```python
from build123d import *

# Parameters (mm, degrees)
EXTRUDE_1_OUTLINE_R   = 35
EXTRUDE_1_OUTLINE_R_2 = 1.55
EXTRUDE_1_OUTLINE_R_3 = 30.05
EXTRUDE_1_DEPTH       = 10
SKETCH_2_R            = 33.525
SKETCH_2_R_2          = 18.525
EXTRUDE_1_2_DEPTH     = 4
SKETCH_3_R            = 1.55
CUT_EXTRUDE_1_DEPTH   = 51.497524692
CUT_EXTRUDE_2_DEPTH   = 6
SKETCH_8_R            = 35
SKETCH_8_R_2          = 30.05
CUT_EXTRUDE_3_DEPTH   = 2
SKETCH_9_R            = 3
CUT_EXTRUDE_4_DEPTH   = 2
SKETCH_10_R           = 1.55
CUT_EXTRUDE_5_DEPTH   = 51.139804547
SKETCH_11_R           = 3
CUT_EXTRUDE_6_DEPTH   = 2
SKETCH_14_R           = 18.525
SKETCH_14_R_2         = 13.5
EXTRUDE_2_DEPTH       = 4
SKETCH_15_R           = 17.5
CUT_EXTRUDE_8_DEPTH   = 1.5
SKETCH_17_R           = 17.5
SKETCH_17_R_2         = 12.5
CUT_EXTRUDE_9_DEPTH   = 1
SKETCH1_R             = 13.5
SKETCH1_R_2           = 12
BOSS_EXTRUDE1_DEPTH   = 1
CUT_EXTRUDE1_START    = -2
SKETCH2_R             = 14
SKETCH2_R_2           = 13.5
CUT_EXTRUDE1_DEPTH    = 2
SKETCH3_R             = 14
SKETCH3_R_2           = 13.6
BOSS_EXTRUDE2_DEPTH   = 2
SKETCH5_R             = 12.5
SKETCH5_R_2           = 12
CUT_EXTRUDE3_DEPTH    = 50.922439844
SKETCH6_R             = 13
SKETCH6_R_2           = 12.5
CUT_EXTRUDE4_DEPTH    = 50.922439844
SKETCH7_R             = 17.5
SKETCH7_R_2           = 13.5
CUT_EXTRUDE5_DEPTH    = 0.5


# Read off the part's stored shape, not the designer's step: 凸台-拉伸1
with BuildPart() as part:
    # Extrude 1 outline → Extrude 1 (new body)
    with BuildSketch(Plane.XY):
        Circle(EXTRUDE_1_OUTLINE_R)
        with Locations((0, -32.5)):
            Circle(EXTRUDE_1_OUTLINE_R_2, mode=Mode.SUBTRACT)
        with Locations((-32.5, 0)):
            Circle(EXTRUDE_1_OUTLINE_R_2, mode=Mode.SUBTRACT)
        Circle(EXTRUDE_1_OUTLINE_R_3, mode=Mode.SUBTRACT)
        with Locations((32.5, 0)):
            Circle(EXTRUDE_1_OUTLINE_R_2, mode=Mode.SUBTRACT)
        with Locations((0, 32.5)):
            Circle(EXTRUDE_1_OUTLINE_R_2, mode=Mode.SUBTRACT)
    extrude(amount=EXTRUDE_1_DEPTH)

    # 草图2 → Extrude 1 2 (add)
    with BuildSketch(Plane.XY.offset(10)):
        Circle(SKETCH_2_R)
        Circle(SKETCH_2_R_2, mode=Mode.SUBTRACT)
    extrude(amount=-EXTRUDE_1_2_DEPTH)

    # 草图3 → 切除-拉伸1 (cut, through all)
    with BuildSketch(Plane(origin=(0, 0, 0), x_dir=(-1, 0, 0), z_dir=(0, 0, -1))):
        with Locations(Location((32.5, 0, 0), (0, 0, 180))):
            Circle(SKETCH_3_R)
        with Locations(Location((0, -32.5, 0), (0, 0, 180))):
            Circle(SKETCH_3_R)
        with Locations(Location((-32.5, 0, 0), (0, 0, 180))):
            Circle(SKETCH_3_R)
        with Locations(Location((0, 32.5, 0), (0, 0, 180))):
            Circle(SKETCH_3_R)
    extrude(amount=-CUT_EXTRUDE_1_DEPTH, mode=Mode.SUBTRACT)

    # 草图7 → 切除-拉伸2 (cut)
    with BuildSketch(Plane(origin=(0, 0, 0), x_dir=(-1, 0, 0), z_dir=(0, 0, -1))):
        with BuildLine():
            Line((15.025, 26.024063384), (17.5, 30.310889132))
            ThreePointArc((17.5, 30.310889132), (24.748737342, 24.748737342), (30.310889132, 17.5))
            Line((30.310889132, 17.5), (26.024063384, 15.025))
            ThreePointArc((26.024063384, 15.025), (21.248558775, 21.248558775), (15.025, 26.024063384))
        make_face()
    extrude(amount=-CUT_EXTRUDE_2_DEPTH, mode=Mode.SUBTRACT)

    # 草图8 → 切除-拉伸3 (cut)
    with BuildSketch(Plane(origin=(0, 0, 0), x_dir=(-1, 0, 0), z_dir=(0, 0, -1))):
        with Locations(Location((0, 0, 0), (0, 0, 30))):
            Circle(SKETCH_8_R)
        Circle(SKETCH_8_R_2, mode=Mode.SUBTRACT)
    extrude(amount=-CUT_EXTRUDE_3_DEPTH, mode=Mode.SUBTRACT)

    # 草图9 → 切除-拉伸4 (cut)
    with BuildSketch(Plane.XY.offset(10)):
        with Locations((0, 32.5)):
            Circle(SKETCH_9_R)
        with Locations((32.5, 0)):
            Circle(SKETCH_9_R)
        with Locations((0, -32.5)):
            Circle(SKETCH_9_R)
        with Locations((-32.5, 0)):
            Circle(SKETCH_9_R)
    extrude(amount=-CUT_EXTRUDE_4_DEPTH, mode=Mode.SUBTRACT)

    # 草图10 → 切除-拉伸5 (cut, through all)
    with BuildSketch(Plane.XY.offset(10)):
        with Locations((22.980970389, 22.980970389)):
            Circle(SKETCH_10_R)
        with Locations((22.980970389, -22.980970389)):
            Circle(SKETCH_10_R)
        with Locations((-22.980970389, -22.980970389)):
            Circle(SKETCH_10_R)
        with Locations((-22.980970389, 22.980970389)):
            Circle(SKETCH_10_R)
    extrude(amount=-CUT_EXTRUDE_5_DEPTH, mode=Mode.SUBTRACT)

    # 草图11 → 切除-拉伸6 (cut)
    with BuildSketch(Plane.XY.offset(10)):
        with Locations((22.980970389, 22.980970389)):
            Circle(SKETCH_11_R)
        with Locations((22.980970389, -22.980970389)):
            Circle(SKETCH_11_R)
        with Locations((-22.980970389, -22.980970389)):
            Circle(SKETCH_11_R)
        with Locations((-22.980970389, 22.980970389)):
            Circle(SKETCH_11_R)
    extrude(amount=-CUT_EXTRUDE_6_DEPTH, mode=Mode.SUBTRACT)

    # 草图14 → 凸台-拉伸2 (add)
    with BuildSketch(Plane.XY.offset(10)):
        Circle(SKETCH_14_R)
        Circle(SKETCH_14_R_2, mode=Mode.SUBTRACT)
    extrude(amount=-EXTRUDE_2_DEPTH)

    # 草图15 → 切除-拉伸8 (cut)
    with BuildSketch(Plane.XY.offset(10)):
        with BuildLine():
            ThreePointArc((21.378493867, 1.75), (0, 21.45), (-21.378493867, 1.75))
            Line((-21.378493866, 1.75), (-24.8, 1.75))
            Line((-24.8, 1.75), (-24.8, -1.75))
            Line((-24.8, -1.75), (-21.378493867, -1.75))
            ThreePointArc((-21.378493867, -1.75), (0, -21.45), (21.378493867, -1.75))
            Line((21.378493867, -1.75), (24.8, -1.75))
            Line((24.8, -1.75), (24.8, 1.75))
            Line((24.8, 1.75), (21.378493867, 1.75))
        make_face()
        Circle(SKETCH_15_R, mode=Mode.SUBTRACT)
    extrude(amount=-CUT_EXTRUDE_8_DEPTH, mode=Mode.SUBTRACT)

    # 草图17 → 切除-拉伸9 (cut)
    with BuildSketch(Plane.XY.offset(10)):
        Circle(SKETCH_17_R)
        Circle(SKETCH_17_R_2, mode=Mode.SUBTRACT)
    extrude(amount=-CUT_EXTRUDE_9_DEPTH, mode=Mode.SUBTRACT)

    # Sketch1 → Boss-Extrude1 (add)
    with BuildSketch(Plane.XY.offset(8.5)):
        Circle(SKETCH1_R)
        Circle(SKETCH1_R_2, mode=Mode.SUBTRACT)
    extrude(amount=-BOSS_EXTRUDE1_DEPTH)

    # Sketch2 → Cut-Extrude1 (cut)
    with BuildSketch(Plane(origin=(0, 0, 6), x_dir=(-1, 0, 0), z_dir=(0, 0, -1)).offset(CUT_EXTRUDE1_START)):
        Circle(SKETCH2_R)
        with Locations(Location((0, 0, 0), (0, 0, 180))):
            Circle(SKETCH2_R_2, mode=Mode.SUBTRACT)
    extrude(amount=CUT_EXTRUDE1_DEPTH, mode=Mode.SUBTRACT)

    # Sketch3 → Boss-Extrude2 (add)
    with BuildSketch(Plane(origin=(0, 0, 7.5), x_dir=(-1, 0, 0), z_dir=(0, 0, -1))):
        Circle(SKETCH3_R)
        Circle(SKETCH3_R_2, mode=Mode.SUBTRACT)
    extrude(amount=BOSS_EXTRUDE2_DEPTH)

    # Sketch5 → Cut-Extrude3 (cut, through all)
    with BuildSketch(Plane.XY.offset(8.5)):
        Circle(SKETCH5_R)
        Circle(SKETCH5_R_2, mode=Mode.SUBTRACT)
    extrude(amount=-CUT_EXTRUDE3_DEPTH, mode=Mode.SUBTRACT)

    # Sketch6 → Cut-Extrude4 (cut, through all)
    with BuildSketch(Plane.XY.offset(8.5)):
        Circle(SKETCH6_R)
        Circle(SKETCH6_R_2, mode=Mode.SUBTRACT)
    extrude(amount=-CUT_EXTRUDE4_DEPTH, mode=Mode.SUBTRACT)

    # Sketch7 → Cut-Extrude5 (cut)
    with BuildSketch(Plane.XY.offset(9)):
        Circle(SKETCH7_R)
        with Locations(Location((0, 0, 0), (0, 0, 180))):
            Circle(SKETCH7_R_2, mode=Mode.SUBTRACT)
    extrude(amount=-CUT_EXTRUDE5_DEPTH, mode=Mode.SUBTRACT)


solid = part.part
```
Source: CAD feature listing. Evaluate the final solid. Frame: model axes, mm. A direction names the side the tool comes from. Round coordinates to 2 decimals unless told otherwise and drop trailing zeros. Loops run counter-clockwise (first coordinate to the right, second up) from the corner with the lowest first, then second, coordinate; pieces in that order, holes last.
(1) Section query D-D (x = -19). Output: boundary loops of the cut face in (y, z), and give its area (3 significant figures).
From the geometry:
outline: (-29.39, 2) - (-23.28, 2) - (-23.28, 6) - (29.39, 6) - (29.39, 10) - (9.96, 10) - (9.96, 8.5) - (-9.96, 8.5) - (-9.96, 10) - (-29.39, 10) - close
area: 230 mm2
(2) Pull-direction query (X, two-part tool) for faces 4 (the flat face through (15, 16, 10)), 5 (the flat face through (-23, -1.75, 9)); classes: +X half, -X half, draft (parallel to the pull), parting line (faces both ways), or undercut.
From the geometry:
face 4: draft
face 5: undercut
(3) Section query A-A (x = -32.5). Output: boundary loops of the cut face in (y, z).
From the geometry:
outline: (-12.99, 2) - (-1.55, 2) - (-1.55, 8) - (-3, 8) - (-3, 10) - (-12.99, 10) - close; (1.55, 2) - (12.99, 2) - (12.99, 10) - (3, 10) - (3, 8) - (1.55, 8) - close
(4) Contact query for flat-ended pins moving along their axis: pin 1 Ø2 at (y, z) = (-19.5, 7) entering from -X; pin 2 Ø1.2 at (y, z) = (0, 9.5) entering from +X; pin 3 Ø1.2 at (y, z) = (0, 9.5) entering from -X; pin 4 Ø2.5 at (x, y) = (22.98, -22.98) entering from -Z. Output: stop coordinate, or through.
From the geometry:
pin 1: stops at x = -29.71
pin 2: stops at x = 29.56
pin 3: stops at x = -29.56
pin 4: passes through
(5) Section query C-C (z = 3). Output: boundary loops of the cut face in (x, y) (3 decimals), and give its area (3 significant figures).
From the geometry:
outline: (-30.311, 17.5) arc R35 ccw (long way) to (-17.5, 30.311) - (-15.025, 26.024) arc R30.05 cw (long way) to (-26.024, 15.025) - close; hole circle Ø3.1 at (-32.5, 0); hole circle Ø3.1 at (-22.981, -22.981); hole circle Ø3.1 at (0, -32.5); hole circle Ø3.1 at (0, 32.5); hole circle Ø3.1 at (22.981, -22.981); hole circle Ø3.1 at (22.981, 22.981); hole circle Ø3.1 at (32.5, 0)
area: 874 mm2
(6) Access query for faces 1 (the cylindrical face through (-31.068, -0.594, 4.958)), 2 (the cylindrical face through (-12.932, -5.362, 5.754)), 3 (the flat face through (21.6, -21.6, 8)). Directions: +Z, -Z, +X, -X, +Y, -Y. A direction counts if a zero-diameter tool reaches every point of the face in a straight line with its end or side. Return the directions, or none.
From the geometry:
face 1: +Z, -Z
face 2: -Z
face 3: +Z
(7) Material intervals for probe 1 along Y at (x, z) = (0, 3.4); probe 2 along X at (y, z) = (-32.5, 5.95); probe 3 along Y at (x, z) = (32.5, 9.25), sorted ascending.
From the geometry:
probe 1: y = -35 to -34.05, -30.95 to -30.05, 30.05 to 30.95, 34.05 to 35
probe 2: x = -12.99 to -1.55, 1.55 to 12.99
probe 3: y = -12.99 to -3, 3 to 12.99
